Here's how the part is built. I have some questions about the finished solid (model axes, mm). A direction names the side the tool comes from. Round coordinates to 2 decimals unless told otherwise and drop trailing zeros. Loops run counter-clockwise (first coordinate to the right, second up) from the corner with the lowest first, then second, coordinate; pieces in that order, holes last. Notation, with made-up numbers: (-29, -30) - (17, -30) arc R29 ccw to (17, -10) - close; hole circle Ø2 at (28.5, 12.5). An arc over 180 degrees is marked (long way). Return JSON: item names as keys, results as strings. Group by question number.
```python
from build123d import *

# Parameters (mm, degrees)
ESBO_O1_W                     = 19
ESBO_O1_H                     = 23
RESSALTO_EXTRUS_O1_DEPTH      = 37
FILETE3_R                     = 4
ESBO_O2_W                     = 3.2
ESBO_O2_H                     = 5.2
RESSALTO_EXTRUS_O2_DEPTH      = 5.030814575
ESBO_O4_R                     = 1.5
CORTE_EXTRUS_O1_DEPTH         = 45.967203313
FILETE4_R                     = 0.5
FILETE5_R                     = 0.5
RESSALTO_EXTRUS_O6_DEPTH      = 9
RESSALTO_EXTRUS_O6_DEPTH_BACK = 28
ESBO_O10_R                    = 2
RESSALTO_EXTRUS_O7_DEPTH      = 2
RESSALTO_EXTRUS_O8_DEPTH      = 11.5
RESSALTO_EXTRUS_O9_DEPTH      = 14
FILETE6_R                     = 2
ESBO_O13_R                    = 5
ESBO_O13_R_2                  = 1
RESSALTO_EXTRUS_O12_DEPTH     = 2.5
FILETE7_R                     = 1.5
ESBO_O14_R                    = 1.5
CORTE_EXTRUS_O2_DEPTH         = 52.796132807
ESBO_O16_R                    = 1.516823529
RESSALTO_EXTRUS_O14_DEPTH     = 7


with BuildPart() as part:
    # Esboço1 → Ressalto-extrusão1 (new body)
    with BuildSketch(Plane(origin=(0, 0, 0), x_dir=(0, 0, -1), z_dir=(1, 0, 0))):
        Rectangle(ESBO_O1_W, ESBO_O1_H)
    extrude(amount=RESSALTO_EXTRUS_O1_DEPTH)

    # Filete3
    filete3_edges = [part.edges().sort_by_distance(p)[0] for p in [
        (37, -11.5, 0),
        (37, 11.5, 0),
    ]]
    fillet(filete3_edges, radius=FILETE3_R)

    # Esboço2 → Ressalto-extrusão2 (add)
    with BuildSketch(Plane(origin=(37, 0, 0), x_dir=(0, 0, -1), z_dir=(1, 0, 0))):
        Rectangle(ESBO_O2_W, ESBO_O2_H)
    extrude(amount=RESSALTO_EXTRUS_O2_DEPTH)

    # Esboço4 → Corte-extrusão1 (cut, through all)
    with BuildSketch(Plane(origin=(0, 0, -1.6), x_dir=(-1, 0, 0), z_dir=(0, 0, -1))):
        with Locations((-39.515407287, 0)):
            Circle(ESBO_O4_R)
    extrude(amount=-CORTE_EXTRUS_O1_DEPTH, mode=Mode.SUBTRACT)

    # Filete4
    filete4_edges = [part.edges().sort_by_distance(p)[0] for p in [
        (37, 2.6, 0),
    ]]
    fillet(filete4_edges, radius=FILETE4_R)

    # Filete5
    filete5_edges = [part.edges().sort_by_distance(p)[0] for p in [
        (37, -2.6, 0),
    ]]
    fillet(filete5_edges, radius=FILETE5_R)

    # Esboço6 → Ressalto-extrusão6 (add, two sides: drawn at the far end of the back side and taken through both)
    with BuildSketch(Plane(origin=(0, 0, -9.5), x_dir=(-1, 0, 0), z_dir=(0, 0, -1)).offset(-RESSALTO_EXTRUS_O6_DEPTH_BACK)):
        with BuildLine():
            Line((-28, -1.887458609), (-28, 1.887458609))
            ThreePointArc((-28, 1.887458609), (-26, 2.75), (-24, 1.887458609))
            Line((-24, 1.887458609), (-24, -1.887458609))
            ThreePointArc((-24, -1.887458609), (-26, -2.75), (-28, -1.887458609))
        make_face()
    extrude(amount=RESSALTO_EXTRUS_O6_DEPTH + RESSALTO_EXTRUS_O6_DEPTH_BACK)

    # Esboço10 → Ressalto-extrusão7 (add)
    with BuildSketch(Plane(origin=(0, 0, -9.5), x_dir=(-1, 0, 0), z_dir=(0, 0, -1))):
        with Locations(Location((-14, 0, 0), (0, 0, 180))):
            Circle(ESBO_O10_R)
    extrude(amount=RESSALTO_EXTRUS_O7_DEPTH)

    # Esboço11 → Ressalto-extrusão8 (add)
    with BuildSketch(Plane.ZY):
        with BuildLine():
            Line((9.5, -7), (9.5, 7))
            ThreePointArc((9.5, 7), (0.75, 11.5), (-8, 7))
            Line((-8, 7), (-8, -7))
            ThreePointArc((-8, -7), (0.75, -11.5), (9.5, -7))
        make_face()
    extrude(amount=RESSALTO_EXTRUS_O8_DEPTH)

    # Esboço12 → Ressalto-extrusão9 (add)
    with BuildSketch(Plane.ZY.offset(11.5)):
        with BuildLine():
            Line((-6.5, 6.498793601), (-6.5, -6.498793601))
            ThreePointArc((-6.5, -6.498793601), (0.75, -10), (8, -6.498793601))
            Line((8, -6.498793601), (8, 6.498793601))
            ThreePointArc((8, 6.498793601), (0.75, 10), (-6.5, 6.498793601))
        make_face()
    extrude(amount=RESSALTO_EXTRUS_O9_DEPTH)

    # Filete6
    filete6_edges = [part.edges().sort_by_distance(p)[0] for p in [
        (-25.5, 10, 0.75),
        (-25.5, 0, -6.5),
        (-25.5, -10, 0.75),
        (-25.5, 0, 8),
    ]]
    fillet(filete6_edges, radius=FILETE6_R)

    # Esboço13 → Ressalto-extrusão12 (add)
    with BuildSketch(Plane.ZY.offset(25.5)):
        with Locations((0.75, 0)):
            Circle(ESBO_O13_R)
        with Locations((0.75, 0)):
            Circle(ESBO_O13_R_2, mode=Mode.SUBTRACT)
    extrude(amount=RESSALTO_EXTRUS_O12_DEPTH)

    # Filete7
    filete7_edges = [part.edges().sort_by_distance(p)[0] for p in [
        (-28, 0, -4.25),
    ]]
    fillet(filete7_edges, radius=FILETE7_R)

    # Esboço14 → Corte-extrusão2 (cut, through all)
    with BuildSketch(Plane(origin=(0, 0, -9.5), x_dir=(-1, 0, 0), z_dir=(0, 0, -1))):
        with Locations((-5.8, 9)):
            Circle(ESBO_O14_R)
        with Locations((-5.8, -9)):
            Circle(ESBO_O14_R)
    extrude(amount=-CORTE_EXTRUS_O2_DEPTH, mode=Mode.SUBTRACT)

    # Esboço16 → Ressalto-extrusão14 (add)
    with BuildSketch(Plane.XY.offset(18.5)):
        with Locations(Location((26, 0, 0), (0, 0, 180))):
            Circle(ESBO_O16_R)
    extrude(amount=RESSALTO_EXTRUS_O14_DEPTH)


solid = part.part
```
Q1. Imagine slicing it at B-B, the plane x = 14. List the corners of the cut face in (y, z) for me.
Q2. Imagine slicing it at A-A, the plane x = 5.8. List the corners of the cut face in (y, z) for me, and give its area (3 significant figures).
Q3. If we mould it in two halves opening along Y, with no side actions, what happens to faces 1 (the cylindrical face through (35.797, -10.359, -0.133)), 2 (the flat face through (0, 0.05, -8.15)), 3 (the cylindrical face through (5.11, -10.33, -0.13))? For each: +Y half, -Y half, draft (parallel to the pull), parting line (faces both ways), or undercut.
Q4. For faces 4 (the flat face through (27.7, 0, 18.5)), 5 (the flat face through (24, 0, 14)), 6 (the flat face through (-25.5, 0, 1)), 7 (the flat face through (14, 0, -11.5)), 8 (the flat face through (24, 0, -14)), which set-ups out of +Z, -Z, +X, -X, +Y, -Y let a thin tool reach every point of the face, with its end or its side?
Q5. Imagine slicing it at C-C, the plane z = 16.5. List the corners of the cut face in (x, y) for me, and give its area (3 significant figures).
Q6. Will these pins go through, and if not, where does the flat tip stop? pin 1 Ø3 at (y, z) = (5.5, -6) entering from -X; pin 2 Ø5.5 at (x, y) = (40.5, -0.5) entering from +Z; pin 3 Ø2.5 at (x, y) = (39.52, 0) entering from +Z; pin 4 Ø13 at (x, y) = (-18.5, -2) entering from -Z.
Q7. Imagine slicing it at D-D, the plane x = 26. List the corners of the cut face in (y, z) for me, and give its area (3 significant figures).
Q8. Please list where these lines run through material, in increasing order: line 1 (Y direction, x = 5.8, z = 3.75); line 2 (Y direction, x = 5, z = 4); line 3 (Z direction, x = -2, y = -1.5).
Output values:
{
 "1": {"outline": "(-11.5, -9.5) - (-2, -9.5) - (-2, -11.5) - (2, -11.5) - (2, -9.5) - (11.5, -9.5) - (11.5, 9.5) - (-11.5, 9.5) - close"},
 "2": {"outline": "(-11.5, -9.5) - (-10.5, -9.5) - (-10.5, 9.5) - (-11.5, 9.5) - close; (-7.5, -9.5) - (7.5, -9.5) - (7.5, 9.5) - (-7.5, 9.5) - close; (10.5, -9.5) - (11.5, -9.5) - (11.5, 9.5) - (10.5, 9.5) - close", "area": "323 mm^2"},
 "3": {"face 1": "-Y half", "face 2": "draft", "face 3": "undercut"},
 "4": {"face 4": "+Z", "face 5": "+Z, -X, +Y, -Y", "face 6": "-X", "face 7": "-Z, -X, +Y, -Y", "face 8": "-Z, +Y, -Y"},
 "5": {"outline": "(24, -1.89) arc R2.75 ccw to (28, -1.89) - (28, 1.89) arc R2.75 ccw to (24, 1.89) - close", "area": "19.9 mm^2"},
 "6": {"pin 1": "stops at x = -25.5", "pin 2": "stops at z = 1.6", "pin 3": "passes through", "pin 4": "stops at z = -6.5"},
 "7": {"outline": "(-11.5, -9.5) - (-2.75, -9.5) - (-2.75, -18.5) - (2.75, -18.5) - (2.75, -9.5) - (11.5, -9.5) - (11.5, 9.5) - (2.75, 9.5) - (2.75, 18.5) - (1.52, 18.5) - (1.52, 25.5) - (-1.52, 25.5) - (-1.52, 18.5) - (-2.75, 18.5) - (-2.75, 9.5) - (-11.5, 9.5) - close", "area": "557 mm^2"},
 "8": {"line 1": "y = -11.5 to -10.5, -7.5 to 7.5, 10.5 to 11.5", "line 2": "y = -11.5 to -10.27, -7.73 to 7.73, 10.27 to 11.5", "line 3": "z = -8 to 9.5"}
}
